Autodesk Inventor part; units mm, degrees
ref_plane "YZ Plane" through (0, 0, 0) normal (1, 0, 0) x (0, 1, 0)
ref_plane "XZ Plane" through (0, 0, 0) normal (0, 1, 0) x (-1, 0, 0)
ref_plane "XY Plane" through (0, 0, 0) normal (0, 0, 1) x (1, 0, 0)
sketch "Sketch1" plane through (0, 0, 0) normal (0, 1, 0) x (-1, 0, 0)
  line L0 (45.25, 31.5) -> (-45.25, 31.5)
  line L1 (-45.25, 31.5) -> (-45.25, -31.5)
  line L2 (-45.25, -31.5) -> (45.25, -31.5)
  line L3 (45.25, -31.5) -> (45.25, 31.5)
  line L4 (45.25, 31.5) -> (-45.25, -31.5) construction
  line L5 (-45.25, 31.5) -> (45.25, -31.5) construction
  point P0 (0, 0)
  dimension "d0" = 63
  dimension "d1" = 90.5
extrude "Extrusion1" add sketch "Sketch1" along normal blind 1.5
sketch "Sketch2" plane through (0, 1.5, 0) normal (0, 1, 0) x (1, 0, 0)
  circle A0 centre (-43.25, -29.5) radius 0.75
  line L0 (-45.25, 31.5) -> (-45.25, -31.5)
  line L1 (-45.25, -31.5) -> (45.25, -31.5)
  circle A1 centre (-43.25, 29.5) radius 0.75
  line L2 (45.25, 31.5) -> (-45.25, 31.5)
  circle A2 centre (43.25, -29.5) radius 0.75
  line L3 (45.25, -31.5) -> (45.25, 31.5)
  circle A3 centre (43.25, 29.5) radius 0.75
  point P0 (0, 0)
  dimension "d4" = 2
  dimension "d5" = 2
  dimension "d6" = 1.5
  dimension "d7" = 2
  dimension "d8" = 2
  dimension "d9" = 1.5
  dimension "d10" = 2
  dimension "d11" = 2
  dimension "d12" = 1.5
  dimension "d13" = 1.5
  dimension "d14" = 2
  dimension "d15" = 2
extrude "Extrusion2" cut sketch "Sketch2" against normal blind 1.5 contours A0 | A1 | A2 | A3
sketch "Sketch6" plane through (0, 1.5, 0) normal (0, 1, 0) x (1, 0, 0)
  line L0 (8.05, -6.1) -> (20.25, -6.1)
  line L1 (20.25, -6.1) -> (20.25, 6.1)
  line L2 (20.25, 6.1) -> (8.05, 6.1)
  line L3 (8.05, 6.1) -> (8.05, -6.1)
  line L4 (-45.25, -31.5) -> (45.25, -31.5)
  line L5 (45.25, -31.5) -> (45.25, 31.5)
  point P0 (0, 0)
  dimension "d42" = 12.2
  dimension "d43" = 12.2
  dimension "d44" = 25.4
  dimension "d45" = 25
extrude "Extrusion6" cut sketch "Sketch6" against normal blind 10
properties part number "remoteswitchlid"
For this review, take the finished solid that the model builds, in its own axes (mm). Give positions to 0.01 mm unless a question says otherwise; leave off trailing zeros. Order: outer loops, then holes, each group sorted by start corner. A loop starts at its lowest first (then second) coordinate and runs counter-clockwise, first axis right, second up.
1) Wall thickness on line 1 (Z direction, x = -43.25, y = 1); line 2 (X direction, y = 0.3, z = -5); line 3 (X direction, y = 0.9, z = 29.5): over which ranges is each line inside the solid? List them lowest first.
2) Insertion check: pin 1 (2 mm diameter, centred on x = -43.25, z = -29.5, fed in from +Y). The pin has a flat end and moves straight along its axis. Give the tip position at first contact, or say it passes through.
3) Take a section at A-A (y = 0.8). Give the boundary of the cut face in (x, z), then the cut area to 3 significant figures.
Derived:
1. line 1: z = -31.5 to -30.25, -28.75 to 28.75, 30.25 to 31.5
1. line 2: x = -45.25 to 8.05, 20.25 to 45.25
1. line 3: x = -45.25 to -44, -42.5 to 42.5, 44 to 45.25
2. pin 1: stops at y = 1.5
3. outline: (-45.25, -31.5) - (45.25, -31.5) - (45.25, 31.5) - (-45.25, 31.5) - close; hole circle Ø1.5 at (-43.25, -29.5); hole circle Ø1.5 at (-43.25, 29.5); hole (8.05, -6.1) - (20.25, -6.1) - (20.25, 6.1) - (8.05, 6.1) - close; hole circle Ø1.5 at (43.25, -29.5); hole circle Ø1.5 at (43.25, 29.5)
3. area: 5,550 mm2
